Input: part model. Units: mm. Frame: model coordinates. A direction names the side the tool comes from. Give positions to 0.01 mm unless a question says otherwise; leave off trailing zeros. Order: outer loops, then holes, each group sorted by start corner. A loop starts at its lowest first (then second) coordinate and runs counter-clockwise, first axis right, second up. Notation, with made-up numbers: (82.25, 64.5) -> (129.25, 64.5) arc R14 ccw to (129.25, 75.5) -> close; hole circle Ø10 at (13, 10.5). An arc over 180 degrees is marked (long way). Use a Markdown table: item, result. Add a question column.
from build123d import *

# Parameters (mm, degrees)
F1_DEPTH  = 22
F3_DEPTH  = 5
F5_DEPTH  = 5
F7_DEPTH  = 25
F8_DEPTH  = 20
F9_W      = 5
F9_H      = 1
F10_DEPTH = 27
F11_W     = 5
F11_H     = 0.5
F12_DEPTH = 1
F13_W     = 5
F13_H     = 0.5
F14_DEPTH = 1


with BuildPart() as f1:
    # F0 (on Front) → F1 (new body)
    with BuildSketch(Plane.XZ):
        with BuildLine():
            ThreePointArc((0, -3.5), (2.4748737342, -2.4748737342), (3.5, 0))
            ThreePointArc((3.5, 0), (2.4748737342, 2.4748737342), (0, 3.5))
            ThreePointArc((0, 3.5), (-2.4748737342, 2.4748737342), (-3.5, 0))
            ThreePointArc((-3.5, 0), (-2.4748737342, -2.4748737342), (0, -3.5))
        make_face()
        with BuildLine():
            ThreePointArc((-3.5, 0), (-2.4748737342, 2.4748737342), (0, 3.5))
            Line((0, 3.5), (-3.5, 3.5))
            Line((-3.5, 3.5), (-3.5, 0))
        make_face()
        with BuildLine():
            Line((-3.5, -3.5), (0, -3.5))
            ThreePointArc((0, -3.5), (-2.4748737342, -2.4748737342), (-3.5, 0))
            Line((-3.5, 0), (-3.5, -3.5))
        make_face()
        with BuildLine():
            Line((3.5, -3.5), (3.5, 0))
            ThreePointArc((3.5, 0), (2.4748737342, -2.4748737342), (0, -3.5))
            Line((0, -3.5), (3.5, -3.5))
        make_face()
        with BuildLine():
            ThreePointArc((0, 3.5), (2.4748737342, 2.4748737342), (3.5, 0))
            Line((3.5, 0), (3.5, 3.5))
            Line((3.5, 3.5), (0, 3.5))
        make_face()
    extrude(amount=F1_DEPTH)

    # F2 (on face) → F3 (join)
    with BuildSketch(Plane.XZ.offset(22)):
        Polygon((3.4641016151, -0.5), (3.4641016151, 0.5), (0, 0.5), (-3.4641016151, 0.5), (-3.4641016151, -0.5), align=None)
    extrude(amount=F3_DEPTH)

    # F4 (on face) → F5 (join)
    with BuildSketch(Plane(origin=(0, 0, 0), x_dir=(-1, 0, 0), z_dir=(0, 1, 0))):
        Polygon((3.4641016151, -0.5), (3.4641016151, 0.5), (0, 0.5), (-3.4641016151, 0.5), (-3.4641016151, -0.5), (0, -0.5), align=None)
    extrude(amount=F5_DEPTH)

    # F6 (on face) → F7 (cut)
    with BuildSketch(Plane(origin=(0, 0, 0), x_dir=(-1, 0, 0), z_dir=(0, 1, 0))):
        with BuildLine():
            ThreePointArc((-3.4641016151, 0.5), (-2.2912878475, 2.6457513111), (0, 3.5))
            Line((0, 3.5), (-3.5, 3.5))
            Line((-3.5, 3.5), (-3.5, 0))
            ThreePointArc((-3.5, 0), (-3.491013868, 0.2506435188), (-3.4641016151, 0.5))
        make_face()
        with BuildLine():
            ThreePointArc((3.4641016151, 0.5), (3.491013868, 0.2506435188), (3.5, 0))
            Line((3.5, 0), (3.5, 3.5))
            Line((3.5, 3.5), (0, 3.5))
            ThreePointArc((0, 3.5), (2.2912878475, 2.6457513111), (3.4641016151, 0.5))
        make_face()
        with BuildLine():
            Line((-3.5, -3.5), (0, -3.5))
            ThreePointArc((0, -3.5), (-2.2912878475, -2.6457513111), (-3.4641016151, -0.5))
            ThreePointArc((-3.4641016151, -0.5), (-3.491013868, -0.2506435188), (-3.5, 0))
            Line((-3.5, 0), (-3.5, -3.5))
        make_face()
        with BuildLine():
            Line((3.5, -3.5), (3.5, 0))
            ThreePointArc((3.5, 0), (3.491013868, -0.2506435188), (3.4641016151, -0.5))
            ThreePointArc((3.4641016151, -0.5), (2.2912878475, -2.6457513111), (0, -3.5))
            Line((0, -3.5), (3.5, -3.5))
        make_face()
    extrude(amount=-F7_DEPTH, mode=Mode.SUBTRACT)

    # F8 (add): a face of the model
    f8_faces = [f1.faces().sort_by_distance(p)[0] for p in [
        (3.4641016151, -24.5, 0),
    ]]
    extrude(f8_faces, amount=F8_DEPTH)

    # F9 (on face) → F10 (join)
    with BuildSketch(Plane(origin=(0, -22, 0), x_dir=(-1, 0, 0), z_dir=(0, 1, 0))):
        with Locations((-20.9641016151, 0)):
            Rectangle(F9_W, F9_H)
    extrude(amount=F10_DEPTH)

    # F11 (on face) → F12 (cut)
    with BuildSketch(Plane(origin=(18.4641016151, 0, 0), x_dir=(0, -1, 0), z_dir=(-1, 0, 0))):
        with Locations((-2.5, 0)):
            Rectangle(F11_W, F11_H)
    extrude(amount=-F12_DEPTH, mode=Mode.SUBTRACT)

    # F13 (on face) → F14 (cut)
    with BuildSketch(Plane.YZ.offset(3.4641016151)):
        with Locations((2.5, 0)):
            Rectangle(F13_W, F13_H)
    extrude(amount=-F14_DEPTH, mode=Mode.SUBTRACT)


solid = f1.part
Q1. Access query for faces 4 (the flat face through (19, 3, -0.25)), 5 (the flat face through (11, -22, 0)), 6 (the flat face through (0, -22, 2)), 7 (the flat face through (-3.464, -24, 0)). Directions: +Z, -Z, +X, -X, +Y, -Y. A direction counts if a zero-diameter tool reaches every point of the face in a straight line with its end or side. Return the directions, or none.
Q2. Section query C-C (x = 15.5). Return loops of the section in (y, z), plus the area to 3 significant figures.
Q3. Draft query along X for faces 1 (the flat face through (3, 2, 0.25)), 2 (the flat face through (0, 0, 2)), 3 (the flat face through (23.464, -11, 0)). Return one class per face: +X half, -X half, draft (parallel to the pull), parting line (faces both ways), or undercut.
Q4. Section query D-D (z = -2.5). Return loops of the section in (x, y).
Q5. Section query A-A (y = 1). Return loops of the section in (x, z), plus the area to 3 significant figures.
Q6. First-contact query: pin 1 (1.1 mm diameter, centred on x = 3, y = 2.5, fed in from -Z); pin 2 (0.8 mm diameter, centred on x = 9, z = 0, fed in from +Y); pin 3 (0.9 mm diameter, centred on x = 0, z = 1.5, fed in from +Y); pin 4 (2.5 mm diameter, centred on x = 1, z = 1.5, fed in from -Y). Flat tips, straight axial feed; report the tip coordinate or a pass-through.
Q7. Ray query, line 1 (X direction, y = -1.5, z = 0.25); line 2 (Y direction, x = -0.25, z = -2.5); line 3 (Y direction, x = 5.5, z = 0.25). Return the intervals inside material, ascending.
Q8. Section query B-B (y = -10). Return loops of the section in (x, z).
Solution:
| question | item | result |
|---|---|---|
| 1 | face 4 | +Y |
| 1 | face 5 | +Z, -Z, +Y |
| 1 | face 6 | +Z, +X, -X, -Y |
| 1 | face 7 | +Z, -Z, -X, -Y |
| 2 | outline | (-27, -0.5) -> (-22, -0.5) -> (-22, 0.5) -> (-27, 0.5) -> close |
| 2 | area | 5.00 mm² |
| 3 | face 1 | undercut |
| 3 | face 2 | draft |
| 3 | face 3 | +X half |
| 4 | outline | (-2.45, -22) -> (2.45, -22) -> (2.45, 0) -> (-2.45, 0) -> close |
| 5 | outline | (-3.46, -0.5) -> (3.46, -0.5) -> (3.46, -0.25) -> (2.46, -0.25) -> (2.46, 0.25) -> (3.46, 0.25) -> (3.46, 0.5) -> (-3.46, 0.5) -> close; (18.46, -0.5) -> (23.46, -0.5) -> (23.46, 0.5) -> (18.46, 0.5) -> (18.46, 0.25) -> (19.46, 0.25) -> (19.46, -0.25) -> (18.46, -0.25) -> close |
| 5 | area | 10.9 mm² |
| 6 | pin 1 | stops at z = -0.5 |
| 6 | pin 2 | stops at y = -22 |
| 6 | pin 3 | stops at y = 0 |
| 6 | pin 4 | stops at y = -27 |
| 7 | line 1 | x = -3.49 to 3.49, 18.46 to 23.46 |
| 7 | line 2 | y = -22 to 0 |
| 7 | line 3 | y = -27 to -22 |
| 8 | outline | circle Ø7 at (0, 0); (18.46, -0.5) -> (23.46, -0.5) -> (23.46, 0.5) -> (18.46, 0.5) -> close |
